```python
from build123d import *

# Parameters (mm, degrees)
SKETCH1_W           = 470
SKETCH1_H           = 20
BOSS_EXTRUDE1_DEPTH = 19.5
SKETCH2_R           = 10
CUT_EXTRUDE1_DEPTH  = 28
LPATTERN1_COUNT     = 8
LPATTERN1_PITCH     = 50
SKETCH3_R           = 2.5
CUT_EXTRUDE2_DEPTH  = 42
SKETCH4_R           = 10
BOSS_EXTRUDE2_DEPTH = 4.8
SKETCH5_R           = 1.5
CUT_EXTRUDE3_DEPTH  = 10


with BuildPart() as part:
    # Sketch1 → Boss-Extrude1 (new, symmetric)
    with BuildSketch(Plane.XY):
        Rectangle(SKETCH1_W, SKETCH1_H)
    extrude(amount=BOSS_EXTRUDE1_DEPTH, both=True)

    # Sketch2 → Cut-Extrude1 (cut)
    with BuildSketch(Plane(origin=(0, 10, 0), x_dir=(1, 0, 0), z_dir=(0, 1, 0))):
        with Locations(Location((-175, 0, 0), (0, 0, 180))):
            Circle(SKETCH2_R)
    cut_extrude1 = extrude(amount=-CUT_EXTRUDE1_DEPTH, mode=Mode.SUBTRACT)

    # LPattern1: Cut-Extrude1 ×8
    with Locations(*[(i * LPATTERN1_PITCH, 0, 0) for i in range(1, LPATTERN1_COUNT)]):
        add(cut_extrude1, mode=Mode.SUBTRACT)

    # Sketch3 → Cut-Extrude2 (cut)
    with BuildSketch(Plane(origin=(0, 10, 0), x_dir=(1, 0, 0), z_dir=(0, 1, 0))):
        with Locations(Location((230, 0, 0), (0, 0, 180))):
            Circle(SKETCH3_R)
    cut_extrude2 = extrude(amount=-CUT_EXTRUDE2_DEPTH, mode=Mode.SUBTRACT)

    # Mirror1: Cut-Extrude2 across plane
    add(cut_extrude2.mirror(Plane(origin=(0, 0, 0), x_dir=(0, 0, 1), z_dir=(1, 0, 0))), mode=Mode.SUBTRACT)

    # Sketch4 → Boss-Extrude2 (add)
    with BuildSketch(Plane(origin=(0, 10, 0), x_dir=(1, 0, 0), z_dir=(0, 1, 0))):
        with Locations(Location((-175, 0, 0), (0, 0, 180))):
            Circle(SKETCH4_R)
        with Locations(Location((-125, 0, 0), (0, 0, 180))):
            Circle(SKETCH4_R)
        with Locations(Location((-75, 0, 0), (0, 0, 180))):
            Circle(SKETCH4_R)
        with Locations(Location((-25, 0, 0), (0, 0, 180))):
            Circle(SKETCH4_R)
        with Locations(Location((25, 0, 0), (0, 0, 180))):
            Circle(SKETCH4_R)
        with Locations(Location((75, 0, 0), (0, 0, 180))):
            Circle(SKETCH4_R)
        with Locations(Location((125, 0, 0), (0, 0, 180))):
            Circle(SKETCH4_R)
        with Locations(Location((175, 0, 0), (0, 0, 180))):
            Circle(SKETCH4_R)
    extrude(amount=-BOSS_EXTRUDE2_DEPTH)

    # Sketch5 → Cut-Extrude3 (cut)
    with BuildSketch(Plane.ZY.offset(235)):
        with Locations((-12.5, 6)):
            Circle(SKETCH5_R)
        with Locations((-12.5, -6)):
            Circle(SKETCH5_R)
        with Locations((9.5, 6)):
            Circle(SKETCH5_R)
        with Locations((9.5, -6)):
            Circle(SKETCH5_R)
    extrude(amount=-CUT_EXTRUDE3_DEPTH, mode=Mode.SUBTRACT)


solid = part.part
```
Verification items for the finished model (mm, model axes). A direction names the side the tool comes from. Coordinates: 2 decimals unless noted, no trailing zeros. Write each loop counter-clockwise with the first axis right and the second up, starting at its lowest first coordinate (ties: lowest second). Pieces come first, ordered by that corner, then holes. Notation, with made-up numbers: M 63.25,-31 L 83.25,-31 A18 ccw 83.25,-24 Z; hole C 32,26.5 d1. An arc over 180 degrees is marked long. Answer as a JSON object with one key per item and string values. Group by question number.
(1) Release check for a two-part mould opening along X. For faces 1 (the face through (-235, 0, 0)), 2 (the face through (135, -2, 0)), 3 (the face through (-3, 0, 19.5)) record: +X half, -X half, draft (parallel to the pull), parting line (faces both ways), or undercut.
(2) Cross-section at C-C, the plane x = 76. Record the cut outline in (y, z), and give its area (3 significant figures).
(3) Material ranges on line 1 (Z direction, x = -125, y = 0); line 2 (Y direction, x = -77, z = -8); line 3 (Z direction, x = -133, y = -7.5), recorded low to high.
(4) Cross-section at A-A, the plane y = -0.75. State how many separate pieces and enclosed holes the cut face has, and give its area (3 significant figures).
(5) Tool access check on faces 4 (the face through (15.763, -2.294, -3.83)), 5 (the face through (-3, -10, 0)). Record the directions out of +Z, -Z, +X, -X, +Y, -Y that give a thin tool (end or side, any length) a straight path to the whole face; none if there is none.
(6) Gauge pin test, flat ends, axial feed: pin 1 (12 mm diameter, centred on x = 25, z = 0, fed in from -Y); pin 2 (0.9 mm diameter, centred on y = -5.5, z = 10, fed in from -X). Record the tip position at first contact, or that the pin passes through.
(7) Cross-section at B-B, the plane x = 125. Record the cut outline in (y, z), and give its area (3 significant figures).
Reply:
{
 "1": {"face 1": "-X half", "face 2": "undercut", "face 3": "draft"},
 "2": {"outline": "M -10,-19.5 L 10,-19.5 L 10,19.5 L -10,19.5 L -10,9.95 L 5.2,9.95 L 5.2,-9.95 L -10,-9.95 Z", "area": "478 mm²"},
 "3": {"line 1": "-19.5 to -10, 10 to 19.5", "line 2": "5.2 to 10", "line 3": "-19.5 to -6, 6 to 19.5"},
 "4": {"separate pieces": "1", "enclosed holes": "10", "area": "15,800 mm²"},
 "5": {"face 4": "-Y", "face 5": "+Z, -Z, +X, -X, -Y"},
 "6": {"pin 1": "y = 5.2", "pin 2": "x = -225"},
 "7": {"outline": "M -10,-19.5 L 10,-19.5 L 10,19.5 L -10,19.5 L -10,10 L 5.2,10 L 5.2,-10 L -10,-10 Z", "area": "476 mm²"}
}
